from build123d import *

# Parameters (mm, degrees)
F0_W      = 35.2
F0_H      = 35.2
F1_DEPTH  = 17.5
F2_SIZE   = 2
F3_R      = 11
F4_DEPTH  = 2
F5_R      = 2
F6_DEPTH  = 5
F7_R      = 2.5
F8_DEPTH  = 19
F10_W     = 5
F10_H     = 19
F11_DEPTH = 15.601


with BuildPart() as f1:
    # F0 (on Top) → F1 (new body, symmetric)
    with BuildSketch(Plane.XY):
        Rectangle(F0_W, F0_H)
    extrude(amount=F1_DEPTH, both=True)

    # F2
    f2_edges = [f1.edges().sort_by_distance(p)[0] for p in [
        (-17.6, 17.6, 0),
        (-17.6, -17.6, 0),
        (17.6, -17.6, 0),
        (17.6, 17.6, 0),
    ]]
    chamfer(f2_edges, length=F2_SIZE)

    # F3 (on face) → F4 (join)
    with BuildSketch(Plane.XY.offset(17.5)):
        Circle(F3_R)
    extrude(amount=F4_DEPTH)

    # F5 (on face) → F6 (cut)
    with BuildSketch(Plane.XY.offset(17.5)):
        with Locations((-13, 13)):
            Circle(F5_R)
        with Locations((13, 13)):
            Circle(F5_R)
        with Locations((-13, -13)):
            Circle(F5_R)
        with Locations((13, -13)):
            Circle(F5_R)
    extrude(amount=-F6_DEPTH, mode=Mode.SUBTRACT)

    # F7 (on face) → F8 (join)
    with BuildSketch(Plane.XY.offset(19.5)):
        Circle(F7_R)
    extrude(amount=F8_DEPTH)

    # F10 (on offset) → F11 (cut, through all)
    with BuildSketch(Plane.XZ.offset(2)):
        with Locations((0, 29)):
            Rectangle(F10_W, F10_H)
    extrude(amount=F11_DEPTH, mode=Mode.SUBTRACT)


solid = f1.part
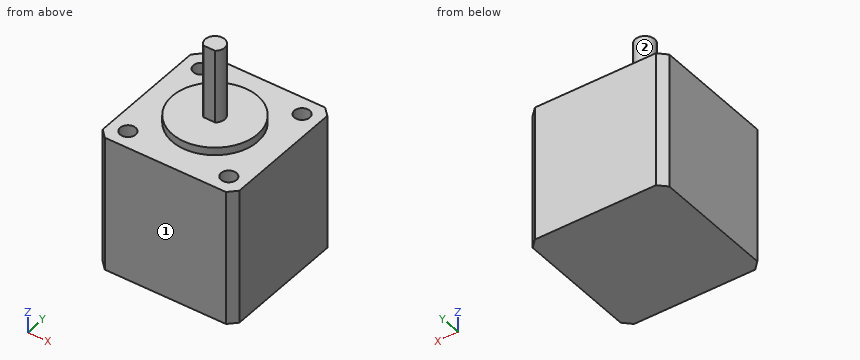
Input: part model. Units: mm. Frame: model coordinates. Face numbers are marked on the shaded views. A direction names the side the tool comes from. Coordinates: 2 decimals unless noted, no trailing zeros. Loops run counter-clockwise (first coordinate to the right, second up) from the corner with the lowest first, then second, coordinate; pieces in that order, holes last.
Q1. Cut plane B-B (y = -13). Output: boundary loops of the cut face in (x, z).
Q2. Cut plane C-C (z = 31). Output: boundary loops of the cut face in (x, y), then the cut area to 3 significant figures.
Q3. Set-up query: the marked faces 1 and 2. Return all of +Z, -Z, +X, -X, +Y, -Y with unobstructed straight access to the full face (end or side cutting, diameter ignored); none if empty.
Q4. Cut plane A-A (x = 0). Output: boundary loops of the cut face in (y, z), then the cut area to 3 significant figures.
Q5. Cut plane D-D (x = 4). Output: boundary loops of the cut face in (y, z), then the cut area to 3 significant figures.
Q6. Contact query for flat-ended pins moving along their axis: pin 1 (2.5 mm diameter, centred on x = 0.5, z = 32.5, fed in from -Y); pin 2 (12 mm diameter, centred on x = 14, z = 29.5, fed in from -Y); pin 3 (3 mm diameter, centred on x = 13, y = -13, fed in from +Z); pin 4 (2 mm diameter, centred on y = 2, z = 24, fed in from -X). Output: stop coordinate, or through.
Q7. Material intervals for line 1 (Y direction, x = 13, z = 14.3); line 2 (Z direction, x = -8.5, y = -4); line 3 (Z direction, x = -12, y = 16.5), sorted ascending.
Working result:
1. outline: (-17.6, -17.5) - (17.6, -17.5) - (17.6, 17.5) - (15, 17.5) - (15, 12.5) - (11, 12.5) - (11, 17.5) - (-11, 17.5) - (-11, 12.5) - (-15, 12.5) - (-15, 17.5) - (-17.6, 17.5) - close
2. outline: (-1.5, -2) - (1.5, -2) arc R2.5 ccw (long way) to start
2. area: 18.6 mm2
3. face 1: +Z, -Z, +X, -X, -Y
3. face 2: +Z
4. outline: (-17.6, -17.5) - (17.6, -17.5) - (17.6, 17.5) - (11, 17.5) - (11, 19.5) - (2.5, 19.5) - (2.5, 38.5) - (-2, 38.5) - (-2, 19.5) - (-11, 19.5) - (-11, 17.5) - (-17.6, 17.5) - close
4. area: 1,360 mm2
5. outline: (-17.6, -17.5) - (17.6, -17.5) - (17.6, 17.5) - (10.25, 17.5) - (10.25, 19.5) - (-10.25, 19.5) - (-10.25, 17.5) - (-17.6, 17.5) - close
5. area: 1,270 mm2
6. pin 1: stops at y = -2
6. pin 2: passes through
6. pin 3: stops at z = 12.5
6. pin 4: stops at x = -2.29
7. line 1: y = -17.6 to -15, -11 to 11, 15 to 17.6
7. line 2: z = -17.5 to 19.5
7. line 3: z = -17.5 to 17.5
